```python
from build123d import *

# Parameters (mm, degrees)
EXTRUSION2_DEPTH           = 161.5
EXTRUSION2_DEPTH_BACK      = 161.5
SKETCH1_R                  = 3.25
F_4_7_4_7_DIAMETER_HOLE1_D = 4.75


with BuildPart() as part:
    # Sketch1 → Extrusion2 (new, two sides: drawn at the far end of the back side and taken through both)
    with BuildSketch(Plane.XY.offset(-EXTRUSION2_DEPTH_BACK)):
        with BuildLine():
            Line((-51.945456549, 19.536039976), (-51.945456549, -0.463960024))
            Line((-51.945456549, -0.463960024), (-49.945456549, -0.463960024))
            Line((-49.945456549, -0.463960024), (-49.945456549, 4.741263919))
            Line((-49.945456549, 4.741263919), (-48.386244669, 4.741263919))
            Line((-48.386244669, 4.741263919), (-43.445456549, -0.1995242))
            Line((-43.445456549, -0.1995242), (-43.445456549, -8.717947961))
            Line((-43.445456549, -8.717947961), (-48.386244669, -13.658736081))
            Line((-48.386244669, -13.658736081), (-49.945456549, -13.658736081))
            Line((-49.945456549, -13.658736081), (-49.945456549, -8.458736081))
            Line((-49.945456549, -8.458736081), (-51.945456549, -8.458736081))
            Line((-51.945456549, -8.458736081), (-51.945456549, -16.458736081))
            ThreePointArc((-51.945456549, -16.458736081), (-51.359670111, -17.872949643), (-49.945456549, -18.458736081))
            Line((-49.945456549, -18.458736081), (-41.945456549, -18.458736081))
            Line((-41.945456549, -18.458736081), (-41.945456549, -16.458736081))
            Line((-41.945456549, -16.458736081), (-47.145456549, -16.458736081))
            Line((-47.145456549, -16.458736081), (-47.145456549, -14.8995242))
            Line((-47.145456549, -14.8995242), (-42.204668429, -9.958736081))
            Line((-42.204668429, -9.958736081), (-33.686244669, -9.958736081))
            Line((-33.686244669, -9.958736081), (-28.745456549, -14.8995242))
            Line((-28.745456549, -14.8995242), (-28.745456549, -16.458736081))
            Line((-28.745456549, -16.458736081), (-33.945456549, -16.458736081))
            Line((-33.945456549, -16.458736081), (-33.945456549, -18.458736081))
            Line((-33.945456549, -18.458736081), (-25.945456549, -18.458736081))
            ThreePointArc((-25.945456549, -18.458736081), (-24.531242987, -17.872949643), (-23.945456549, -16.458736081))
            Line((-23.945456549, -16.458736081), (-23.945456549, -8.458736081))
            Line((-23.945456549, -8.458736081), (-25.945456549, -8.458736081))
            Line((-25.945456549, -8.458736081), (-25.945456549, -13.658736081))
            Line((-25.945456549, -13.658736081), (-27.504668429, -13.658736081))
            Line((-27.504668429, -13.658736081), (-32.445456549, -8.717947961))
            Line((-32.445456549, -8.717947961), (-32.445456549, -0.1995242))
            Line((-32.445456549, -0.1995242), (-27.504668429, 4.741263919))
            Line((-27.504668429, 4.741263919), (-25.945456549, 4.741263919))
            Line((-25.945456549, 4.741263919), (-25.945456549, -0.463960024))
            Line((-25.945456549, -0.463960024), (-23.945456549, -0.463960024))
            Line((-23.945456549, -0.463960024), (-23.945456549, 19.541263919))
            Line((-23.945456549, 19.541263919), (-25.945456549, 19.541263919))
            Line((-25.945456549, 19.541263919), (-25.945456549, 14.341263919))
            Line((-25.945456549, 14.341263919), (-27.504668429, 14.341263919))
            Line((-27.504668429, 14.341263919), (-32.445456549, 19.282052039))
            Line((-32.445456549, 19.282052039), (-32.445456549, 27.8004758))
            Line((-32.445456549, 27.8004758), (-27.504668429, 32.741263919))
            Line((-27.504668429, 32.741263919), (-25.945456549, 32.741263919))
            Line((-25.945456549, 32.741263919), (-25.945456549, 27.541263919))
            Line((-25.945456549, 27.541263919), (-23.945456549, 27.541263919))
            Line((-23.945456549, 27.541263919), (-23.945456549, 35.541263919))
            ThreePointArc((-23.945456549, 35.541263919), (-24.531242987, 36.955477482), (-25.945456549, 37.541263919))
            Line((-25.945456549, 37.541263919), (-33.945456549, 37.541263919))
            Line((-33.945456549, 37.541263919), (-33.945456549, 35.541263919))
            Line((-33.945456549, 35.541263919), (-28.745456549, 35.541263919))
            Line((-28.745456549, 35.541263919), (-28.745456549, 33.982052039))
            Line((-28.745456549, 33.982052039), (-33.686244669, 29.041263919))
            Line((-33.686244669, 29.041263919), (-42.204668429, 29.041263919))
            Line((-42.204668429, 29.041263919), (-47.145456549, 33.982052039))
            Line((-47.145456549, 33.982052039), (-47.145456549, 35.541263919))
            Line((-47.145456549, 35.541263919), (-41.945456549, 35.541263919))
            Line((-41.945456549, 35.541263919), (-41.945456549, 37.541263919))
            Line((-41.945456549, 37.541263919), (-49.945456549, 37.541263919))
            ThreePointArc((-49.945456549, 37.541263919), (-51.359670111, 36.955477482), (-51.945456549, 35.541263919))
            Line((-51.945456549, 35.541263919), (-51.945456549, 27.541263919))
            Line((-51.945456549, 27.541263919), (-49.945456549, 27.541263919))
            Line((-49.945456549, 27.541263919), (-49.945456549, 32.736039976))
            Line((-49.945456549, 32.736039976), (-48.372120999, 32.736039976))
            Line((-48.372120999, 32.736039976), (-43.43133288, 27.795251856))
            Line((-43.43133288, 27.795251856), (-43.43133288, 19.276828096))
            Line((-43.43133288, 19.276828096), (-48.372120999, 14.336039976))
            Line((-48.372120999, 14.336039976), (-49.93133288, 14.336039976))
            Line((-49.93133288, 14.336039976), (-49.93133288, 19.536039976))
            Line((-49.93133288, 19.536039976), (-51.945456549, 19.536039976))
        make_face()
        with Locations((-37.945456549, -4.458736081)):
            Circle(SKETCH1_R, mode=Mode.SUBTRACT)
        with Locations((-37.945456549, 23.541263919)):
            Circle(SKETCH1_R, mode=Mode.SUBTRACT)
        Polygon((-33.686244669, 18.041263919), (-42.204668429, 18.041263919), (-47.145456549, 13.1004758), (-47.145456549, 5.982052039), (-42.204668429, 1.041263919), (-33.686244669, 1.041263919), (-28.745456549, 5.982052039), (-28.745456549, 13.1004758), align=None, mode=Mode.SUBTRACT)
    extrude(amount=EXTRUSION2_DEPTH + EXTRUSION2_DEPTH_BACK)

    # Ø4.7 (4.7) Diameter Hole1 (through all)
    with Locations(Plane(origin=(-23.945456549, 0, 0), x_dir=(0, 0, -1), z_dir=(1, 0, 0))):
        with Locations((-140.5, 23.541263919), (140.5, 23.541263919)):
            Hole(F_4_7_4_7_DIAMETER_HOLE1_D / 2)


solid = part.part
```
Here's how the part is built. I have some questions about the finished solid (model axes, mm). A direction names the side the tool comes from. Round coordinates to 2 decimals unless told otherwise and drop trailing zeros. Write each loop counter-clockwise with the first axis right and the second up, starting at its lowest first coordinate (ties: lowest second). Pieces come first, ordered by that corner, then holes. Notation, with made-up numbers: M 88.25,-23.5 L 146.25,-23.5 A25 cw 146.25,-5.5 Z; hole C 83,12.5 d7. An arc over 180 degrees is marked long. Answer as CSV lines item,"result". Start each with the question number.
1. I'm going to push flat-ended pins straight in: pin 1 Ø1.6 at (y, z) = (36, -35) entering from -X; pin 2 Ø0.6 at (y, z) = (36, -51) entering from +X; pin 3 Ø1 at (x, z) = (-51.5, -55) entering from -Y; pin 4 Ø3 at (y, z) = (23.54, 140.5) entering from -X. Where does each tip first touch, or does it pass through?
2. Thinking about a two-plate mould opening in Y: for faces 1 (the flat face through (-51.945, -12, -2)), 2 (the flat face through (-43.445, -4, -2)), which applies, released by +Y, released by -Y, zero draft, split by the parting line, or undercut?
3. On a 3-axis mill with a long thin cutter (end or side, diameter ignored), from which of +Z, -Z, +X, -X, +Y, -Y can I reach the whole of each face in a straight line? I mean faces 3 (the flat face through (-29.94, -11.223, -2.261)), 4 (the flat face through (-51.945, 10, -2)). Say none if no direction works.
4. I need wall thicknesses on probe 1 along Y at (x, z) = (-50, -2); probe 2 along Y at (x, z) = (-27.25, 65); probe 3 along Y at (x, z) = (-37.5, 122.5). Which ranges of each line are inside material? Lowest first, please.
5. Suppose I cut it at B-B on z = -70. Count the separate pieces of the cut face and the enclosed holes in it, then the cut area to 3 significant figures.
6. Suppose I cut it at A-A on y = 9. Write out the boundary of the cut face in (x, z).
Check result:
1,pin 1,"stops at x = -51.95"
1,pin 2,"stops at x = -23.95"
1,pin 3,"stops at y = -18.16"
1,pin 4,"passes through"
2,face 1,"zero draft"
2,face 2,"undercut"
3,face 3,"+Z, -Z"
3,face 4,"+Z, -Z, -X, +Y, -Y"
4,probe 1,"y = -18.46 to -8.46, -0.46 to 19.54, 27.54 to 37.54"
4,probe 2,"y = -18.46 to -13.66, 4.74 to 14.34, 32.74 to 37.54"
4,probe 3,"y = -9.96 to -7.68, -1.24 to 1.04, 18.04 to 20.32, 26.76 to 29.04"
5,separate pieces,"1"
5,enclosed holes,"3"
5,area,"567 mm2"
6,outline,"M -51.95,-161.5 L -47.15,-161.5 L -47.15,161.5 L -51.95,161.5 Z; M -28.75,-161.5 L -23.95,-161.5 L -23.95,161.5 L -28.75,161.5 Z"
